Part model, mm, in its own coordinate system. Face numbers are marked on the shaded views. A direction names the side the tool comes from. Give positions to 0.01 mm unless a question says otherwise; leave off trailing zeros. Write each loop counter-clockwise with the first axis right and the second up, starting at its lowest first coordinate (ties: lowest second). Pieces come first, ordered by that corner, then holes. Notation, with made-up numbers: M 76,-34.5 L 103,-34.5 A28 cw 103,-8.5 Z; hole C 44,-21.75 d7. An arc over 180 degrees is marked long. Answer as CSV lines item,"result". Start each with the question number.
Item 1: Band-saw the part on C-C, the plane y = 34. List the corners of the cut face in (x, z), then the cut area to 3 significant figures.
Item 2: 3-axis set-ups, long thin cutter, end or side, ignore diameter. For the marked faces 4 and 5: which of +Z, -Z, +X, -X, +Y, -Y reach the whole face in a straight line?
Item 3: Band-saw the part on A-A, the plane x = 0. List the corners of the cut face in (y, z).
Item 4: Pin check, flat tips, straight feed: pin 1 (16.5 mm diameter, centred on x = 0, y = 0, fed in from +Z); pin 2 (2 mm diameter, centred on y = -5, z = 12, fed in from +X); pin 3 (1 mm diameter, centred on x = 22, z = 22.5, fed in from +Y); pin 4 (10 mm diameter, centred on x = -28, z = 18, fed in from +Y). Stop position of each tip, or through.
Item 5: Band-saw the part on D-D, the plane z = 23. List the corners of the cut face in (x, y).
Item 6: Wall check: L1, parallel to Y at x = 0.5, z = 3; L2, parallel to Z at x = -34, y = 1; L3, parallel to Z at x = 15.5, y = 26. Give the ranges that are in metal, low to high. Write a range as from..to.
Item 7: Two-plate mould, pull along X, no slides. Class the marked faces 1, 2 and 3: +X half, -X half, draft (parallel to the pull), parting line (faces both ways), or undercut.
from build123d import *

# Parameters (mm, degrees)
F0_W     = 86.106
F0_H     = 86.106
F1_DEPTH = 10.922
F3_D     = 11.43
F5_DEPTH = 14.478
F5_TAPER = 5
F6_R     = 12.7
F7_DEPTH = 7.874
F9_D     = 12.7
F10_R    = 5.5245


with BuildPart() as f1:
    # F0 (on Top) → F1 (new body)
    with BuildSketch(Plane.XY):
        Rectangle(F0_W, F0_H)
    extrude(amount=F1_DEPTH)

    # F3 (through all)
    with Locations(Plane.XY.offset(10.922)):
        with Locations((-32.004, 32.004), (32.004, 32.004), (32.004, -32.004), (-32.004, -32.004)):
            Hole(F3_D / 2)

    # F4 (on face) → F5 (join)
    with BuildSketch(Plane.XY.offset(10.922)):
        with BuildLine():
            ThreePointArc((32.004, 0), (22.6302453978, 22.6302454524), (-7.72e-08, 32.004))
            ThreePointArc((-7.72e-08, 32.004), (-22.6302453978, -22.6302454524), (32.004, 0))
        make_face()
    extrude(amount=F5_DEPTH, taper=F5_TAPER)

    # F6 (on face) → F7 (join)
    with BuildSketch(Plane.XY.offset(25.4)):
        Circle(F6_R)
    extrude(amount=F7_DEPTH)

    # F9 (through all)
    with Locations(Plane.XY.offset(33.274)):
        with Locations((0, 0)):
            Hole(F9_D / 2)

    # F10
    f10_edges = [f1.edges().sort_by_distance(p)[0] for p in [
        (43.053, 43.053, 5.461),
        (43.053, -43.053, 5.461),
        (-43.053, -43.053, 5.461),
        (-43.053, 43.053, 5.461),
    ]]
    fillet(f10_edges, radius=F10_R)


solid = f1.part
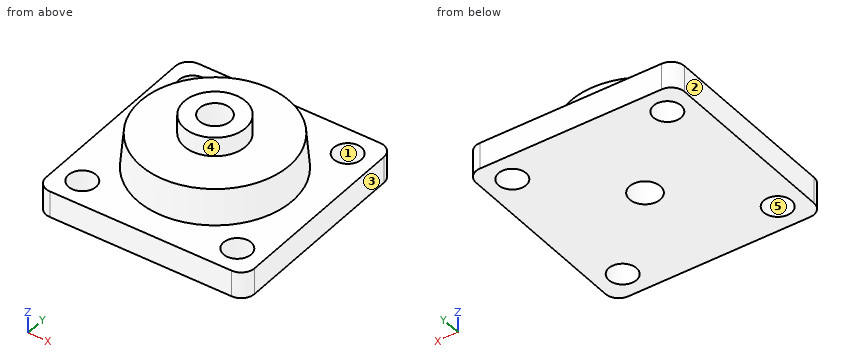
Output:
1,outline,"M -43.05,0 L -37.36,0 L -37.36,10.92 L -43.05,10.92 Z; M -26.65,0 L 26.65,0 L 26.65,10.92 L -26.65,10.92 Z; M 37.36,0 L 43.05,0 L 43.05,10.92 L 37.36,10.92 Z"
1,area,"706 mm²"
2,face 4,"+Z"
2,face 5,"+Z, -Z"
3,outline,"M -43.05,0 L -6.35,0 L -6.35,33.27 L -12.7,33.27 L -12.7,25.4 L -30.74,25.4 L -32,10.92 L -43.05,10.92 Z; M 6.35,0 L 43.05,0 L 43.05,10.92 L 32,10.92 L 30.74,25.4 L 12.7,25.4 L 12.7,33.27 L 6.35,33.27 Z"
4,pin 1,"z = 33.27"
4,pin 2,"x = 31.69"
4,pin 3,"y = 22.32"
4,pin 4,"y = 21.39"
5,outline,"C 0,0 d61.89; hole C 0,0 d12.7"
6,L1,"-43.05..-6.33, 6.33..43.05"
6,L2,"0..10.92"
6,L3,"0..25.4"
7,face 1,"undercut"
7,face 2,"-X half"
7,face 3,"+X half"
